Build history of the part. All positions in model axes, mm. A direction names the side the tool comes from. Give positions to 0.01 mm unless a question says otherwise; leave off trailing zeros. Order: outer loops, then holes, each group sorted by start corner. A loop starts at its lowest first (then second) coordinate and runs counter-clockwise, first axis right, second up. Notation, with made-up numbers: M -27.5,-37 L 13.5,-37 A14 cw 13.5,-11 Z; hole C 55,-3.75 d1. An arc over 180 degrees is marked long. Answer as CSV lines item,"result".
from build123d import *

# Parameters (mm, degrees)
SKETCH1_R           = 2.413
SKETCH1_R_2         = 0.75
BOSS_EXTRUDE1_DEPTH = 2


with BuildPart() as part:
    # Sketch1 → Boss-Extrude1 (new, symmetric)
    with BuildSketch(Plane(origin=(0, 0, 0), x_dir=(0, 0, -1), z_dir=(1, 0, 0))):
        Polygon((-40.864531886, 18.395870563), (-43.06614877, 6.35), (-43.06614877, -6.35), (-6.35, -6.35), (-6.35, -43.06614877), (6.35, -43.06614877), (6.35, 6.35), (-12.928006667, 6.35), (-26.539165493, 15.777631529), align=None)
        Circle(SKETCH1_R, mode=Mode.SUBTRACT)
        with Locations((3.481818182, -38.06614877)):
            Circle(SKETCH1_R_2, mode=Mode.SUBTRACT)
        with Locations((1.336363636, -38.06614877)):
            Circle(SKETCH1_R_2, mode=Mode.SUBTRACT)
        with Locations((-5.1, -38.06614877)):
            Circle(SKETCH1_R_2, mode=Mode.SUBTRACT)
        with Locations((-2.954545455, -38.06614877)):
            Circle(SKETCH1_R_2, mode=Mode.SUBTRACT)
        with Locations((-0.809090909, -38.06614877)):
            Circle(SKETCH1_R_2, mode=Mode.SUBTRACT)
    extrude(amount=BOSS_EXTRUDE1_DEPTH, both=True)


solid = part.part
Item 1: Probe line 1 along Y through (x, z) = (0.9, 0); line 2 along Y through (x, z) = (0.3, -1); line 3 along Z through (x, y) = (1.35, -11.5). List the from-to ranges inside material, lowest first. Write a range as from..to.
Geometry says:
line 1,"y = -43.07..-2.41, 2.41..6.35"
line 2,"y = -43.07..-38.74, -37.4..-2.2, 2.2..6.35"
line 3,"z = -6.35..6.35"
Item 2: Band-saw the part on A-A (z = 5.1). Give the cut face in (x, y).
Geometry says:
outline,"M -2,-43.07 L 2,-43.07 L 2,-38.82 L -2,-38.82 Z; M -2,-37.32 L 2,-37.32 L 2,6.35 L -2,6.35 Z"
Item 3: Drop flat-ended pins along their axis: pin 1 (1.4 mm diameter, centred on y = -38.07, z = -3.48, fed in from -X); pin 2 (1.2 mm diameter, centred on x = 1, y = -30.5, fed in from +Z); pin 3 (2 mm diameter, centred on x = 0.5, z = 2, fed in from +Y). Give the stop position or say it passes through.
Geometry says:
pin 1,"passes through"
pin 2,"stops at z = 6.35"
pin 3,"stops at y = 6.35"
Item 4: Band-saw the part on C-C (x = 1). Give the cut face in (y, z).
Geometry says:
outline,"M -43.07,-6.35 L 6.35,-6.35 L 6.35,12.93 L 15.78,26.54 L 18.4,40.86 L 6.35,43.07 L -6.35,43.07 L -6.35,6.35 L -43.07,6.35 Z; hole C -38.07,-3.48 d1.5; hole C -38.07,-1.34 d1.5; hole C -38.07,0.81 d1.5; hole C -38.07,2.95 d1.5; hole C -38.07,5.1 d1.5; hole C 0,0 d4.83"
Item 5: Pull direction Z, two halves, no side cores. Call faces 1 (the flat face through (0.03, 12.46, 41.95)), 2 (the cylindrical face through (-0.03, -38.73, 0.46)), 3 (the flat face through (0, -19, -6.35)), 4 (the flat face through (0, 6.35, 3)): released by +Z, released by -Z, zero draft, split by the parting line, or undercut.
Geometry says:
face 1,"released by +Z"
face 2,"undercut"
face 3,"released by -Z"
face 4,"zero draft"
Item 6: Band-saw the part on B-B (y = 0). Give the cut face in (x, z).
Geometry says:
outline,"M -2,-6.35 L 2,-6.35 L 2,-2.41 L -2,-2.41 Z; M -2,2.41 L 2,2.41 L 2,43.07 L -2,43.07 Z"
Item 7: Band-saw the part on D-D (z = 27.5). Give the cut face in (x, y), and give its area (3 significant figures).
Geometry says:
outline,"M -2,-6.35 L 2,-6.35 L 2,15.95 L -2,15.95 Z"
area,"89.2 mm2"
Item 8: 3-axis set-ups, long thin cutter, end or side, ignore diameter. For faces 5 (the flat face through (0, -24, 6.35)), 6 (the cylindrical face through (-0.03, -38.73, 4.75)): which of +Z, -Z, +X, -X, +Y, -Y reach the whole face in a straight line?
Geometry says:
face 5,"+Z, +X, -X, -Y"
face 6,"+X, -X"
